Could you check a few things on this model? Use its own coordinates, in mm. Face numbers are marked on the shaded views. A direction names the side the tool comes from. Give positions to 0.01 mm unless a question says otherwise; leave off trailing zeros. Order: outer loops, then holes, each group sorted by start corner. A loop starts at its lowest first (then second) coordinate and runs counter-clockwise, first axis right, second up.
(1) Imagine slicing it at A-A, the plane z = 0. Write out the boundary of the cut face in (x, y), then the cut area to 3 significant figures.
(2) If we mould it in two halves opening along X, with no side actions, what happens to the marked faces 1, 2 and 3? For each: released by +X, released by -X, zero draft, split by the parting line, or undercut.
(3) If I drill on probe 1 along Z at (x, y) = (218.75, -113.75); probe 2 along Y at (x, z) = (218.5, 0); probe 3 along X at (y, z) = (-105.75, 1), over which ranges is the centre line in solid material (lowest first)?
(4) On a 3-axis mill with a long thin cutter (end or side, diameter ignored), from which of +Z, -Z, +X, -X, +Y, -Y can I reach the whole of each face in a straight line? I mean the marked faces 4 and 5. Say none if no direction works.
(5) Imagine slicing it at B-B, the plane x = 219.75. Write out the boundary of the cut face in (y, z).
(6) Will these pins go through, and if not, where does the flat tip stop? pin 1 (3 mm diameter, centred on x = 222, z = -5, fed in from +Y); pin 2 (2 mm diameter, centred on x = 218.5, y = -111.5, fed in from +Z); pin 3 (11 mm diameter, centred on y = -113.68, z = 0, fed in from +X); pin 4 (1 mm diameter, centred on x = 221, y = -112.5, fed in from -Z).
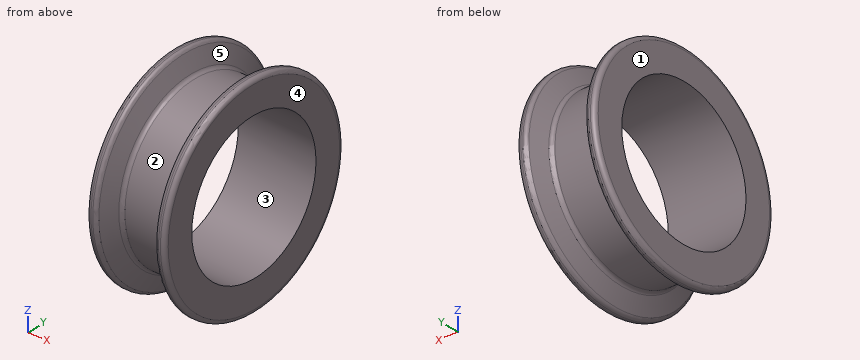
from build123d import *


with BuildPart() as part:
    # Sketch1 → Revolve1 (revolve)
    with BuildSketch(Plane.XY, mode=Mode.PRIVATE) as revolve1_sk:
        with BuildLine():
            Line((215.569737887, -120.531915067), (223.024189817, -120.531915067))
            Line((223.024189817, -120.531915067), (223.024189817, -123.131915067))
            ThreePointArc((223.024189817, -123.131915067), (222.90703253, -123.41475778), (222.624189817, -123.531915067))
            Line((222.624189817, -123.531915067), (222.453461469, -123.531915067))
            ThreePointArc((222.453461469, -123.531915067), (222.22974276, -123.463502069), (222.08255039, -123.281664764))
            Line((222.08255039, -123.281664764), (221.477150355, -121.78216537))
            ThreePointArc((221.477150355, -121.78216537), (221.329957985, -121.600328066), (221.106239276, -121.531915067))
            Line((221.106239276, -121.531915067), (217.487688428, -121.531915067))
            ThreePointArc((217.487688428, -121.531915067), (217.26396972, -121.600328066), (217.11677735, -121.78216537))
            Line((217.11677735, -121.78216537), (216.511377314, -123.281664764))
            ThreePointArc((216.511377314, -123.281664764), (216.364184944, -123.463502069), (216.140466236, -123.531915067))
            Line((216.140466236, -123.531915067), (215.969737887, -123.531915067))
            ThreePointArc((215.969737887, -123.531915067), (215.686895175, -123.41475778), (215.569737887, -123.131915067))
            Line((215.569737887, -123.131915067), (215.569737887, -120.531915067))
        make_face()
    revolve(revolve1_sk.sketch.rotate(Axis((220.434983076, -113.681915067, 0), (-1, 0, 0)), 270), axis=Axis((220.434983076, -113.681915067, 0), (-1, 0, 0)))


solid = part.part
Answer block:
1. outline: (215.57, -123.13) arc R0.4 ccw to (215.97, -123.53) - (216.14, -123.53) arc R0.4 ccw to (216.51, -123.28) - (217.12, -121.78) arc R0.4 cw to (217.49, -121.53) - (221.11, -121.53) arc R0.4 cw to (221.48, -121.78) - (222.08, -123.28) arc R0.4 ccw to (222.45, -123.53) - (222.62, -123.53) arc R0.4 ccw to (223.02, -123.13) - (223.02, -120.53) - (215.57, -120.53) - close; (215.57, -106.83) - (223.02, -106.83) - (223.02, -104.23) arc R0.4 ccw to (222.62, -103.83) - (222.45, -103.83) arc R0.4 ccw to (222.08, -104.08) - (221.48, -105.58) arc R0.4 cw to (221.11, -105.83) - (217.49, -105.83) arc R0.4 cw to (217.12, -105.58) - (216.51, -104.08) arc R0.4 ccw to (216.14, -103.83) - (215.97, -103.83) arc R0.4 ccw to (215.57, -104.23) - close
1. area: 24.7 mm2
2. face 1: released by -X
2. face 2: undercut
2. face 3: zero draft
3. probe 1: z = -7.85 to -6.85, 6.85 to 7.85
3. probe 2: y = -121.53 to -120.53, -106.83 to -105.83
3. probe 3: x = 215.57 to 217.18, 221.41 to 223.02
4. face 4: +Z, -Z, +X, +Y, -Y
4. face 5: none
5. outline: circle Ø15.7 at (-113.68, 0); hole circle Ø13.7 at (-113.68, 0)
6. pin 1: stops at y = -104.5
6. pin 2: stops at z = 7.76
6. pin 3: passes through
6. pin 4: stops at z = -8.07
